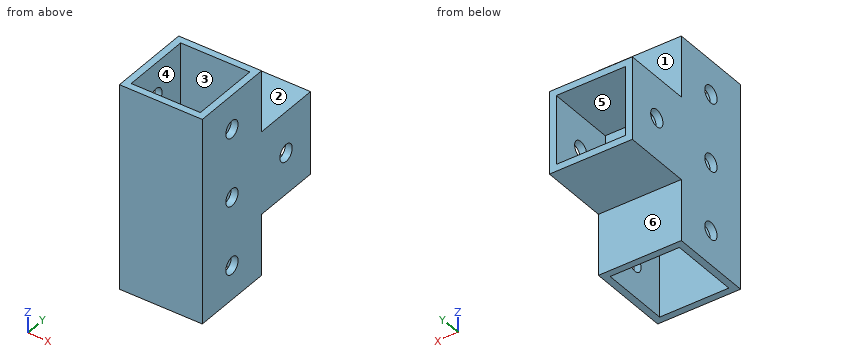
from build123d import *

# Parameters (mm, degrees)
SKETCH_2_W          = 24.2
SKETCH_2_H          = 24.2
SKETCH_2_W_2        = 20.2
SKETCH_2_H_2        = 20.2
EXTRUDE_4_DEPTH     = 100
SKETCH_6_W          = 24.2
SKETCH_6_H          = 24.2
SKETCH_6_W_2        = 20.2
SKETCH_6_H_2        = 20.2
EXTRUDE_5_DEPTH     = 40
SKETCH_7_R          = 2.5
CUT_EXTRUDE_1_DEPTH = 40
SKETCH_8_R          = 2.5
CUT_EXTRUDE_2_DEPTH = 40
CUT_EXTRUDE_START   = -40
SKETCH_9_W          = 20
SKETCH_9_H          = 24.2
SKETCH_9_R          = 2.5
CUT_EXTRUDE_3_DEPTH = 40
SKETCH_10_W         = 24.2
SKETCH_10_H         = 20
SKETCH_10_R         = 2.5
CUT_EXTRUDE_4_DEPTH = 40


with BuildPart() as part:
    # 草图2 → 凸台-拉伸4 (new body)
    with BuildSketch(Plane.XY):
        Rectangle(SKETCH_2_W, SKETCH_2_H)
        Rectangle(SKETCH_2_W_2, SKETCH_2_H_2, mode=Mode.SUBTRACT)
    extrude(amount=EXTRUDE_4_DEPTH)

    # 草图6 → 凸台-拉伸5 (add)
    with BuildSketch(Plane(origin=(0, 12.1, 0), x_dir=(1, 0, 0), z_dir=(0, 1, 0))):
        with Locations((0, -50)):
            Rectangle(SKETCH_6_W, SKETCH_6_H)
        with Locations((0, -50)):
            Rectangle(SKETCH_6_W_2, SKETCH_6_H_2, mode=Mode.SUBTRACT)
    extrude(amount=EXTRUDE_5_DEPTH)

    # 草图7 → 切除-拉伸1 (cut)
    with BuildSketch(Plane.ZY.offset(12.1)):
        with Locations((10, 0)):
            Circle(SKETCH_7_R)
        with Locations((30, 0)):
            Circle(SKETCH_7_R)
        with Locations(Location((90, 0, 0), (0, 0, 180))):
            Circle(SKETCH_7_R)
        with Locations(Location((70, 0, 0), (0, 0, 180))):
            Circle(SKETCH_7_R)
        with Locations((50, 42.1)):
            Circle(SKETCH_7_R)
        with Locations((50, 22.1)):
            Circle(SKETCH_7_R)
    extrude(amount=-CUT_EXTRUDE_1_DEPTH, mode=Mode.SUBTRACT)

    # 草图8 → 切除-拉伸2 (cut)
    with BuildSketch(Plane(origin=(12.1, 0, 0), x_dir=(0, 0, -1), z_dir=(1, 0, 0))):
        with Locations((-50, 0)):
            Circle(SKETCH_8_R)
    extrude(amount=-CUT_EXTRUDE_2_DEPTH, mode=Mode.SUBTRACT)

    # 草图9 → 切除-拉伸3 (cut)
    # profile 1 of 2: a face of its own
    with BuildSketch(Plane(origin=(12.1, 0, 0), x_dir=(0, 0, -1), z_dir=(1, 0, 0)).offset(CUT_EXTRUDE_START)):
        with Locations((-10, 0)):
            Rectangle(SKETCH_9_W, SKETCH_9_H)
        with Locations((-10, 0)):
            Circle(SKETCH_9_R, mode=Mode.SUBTRACT)
    # profile 2 of 2: a face of its own
    with BuildSketch(Plane(origin=(12.1, 0, 0), x_dir=(0, 0, -1), z_dir=(1, 0, 0)).offset(CUT_EXTRUDE_START)):
        with Locations((-90, 0)):
            Rectangle(SKETCH_9_W, SKETCH_9_H)
        with Locations((-90, 0)):
            Circle(SKETCH_9_R, mode=Mode.SUBTRACT)
    extrude(amount=CUT_EXTRUDE_3_DEPTH, mode=Mode.SUBTRACT)

    # 草图10 → 切除-拉伸4 (cut)
    with BuildSketch(Plane(origin=(12.1, 0, 0), x_dir=(0, 0, -1), z_dir=(1, 0, 0)).offset(CUT_EXTRUDE_START)):
        with Locations((-50, 42.1)):
            Rectangle(SKETCH_10_W, SKETCH_10_H)
        with Locations((-50, 42.1)):
            Circle(SKETCH_10_R, mode=Mode.SUBTRACT)
    extrude(amount=CUT_EXTRUDE_4_DEPTH, mode=Mode.SUBTRACT)


solid = part.part
Source: CAD feature listing. Evaluate the final solid. Frame: model axes, mm. Face numbers are marked on the shaded views. A direction names the side the tool comes from. Round coordinates to 2 decimals unless told otherwise and drop trailing zeros. Write each loop counter-clockwise with the first axis right and the second up, starting at its lowest first coordinate (ties: lowest second). Pieces come first, ordered by that corner, then holes. Notation, with made-up numbers: M -20.5,-15 L 8.5,-15 A18 ccw 8.5,-1 Z; hole C 42,83.25 d6. An arc over 180 degrees is marked long. One line per item, written item: value. Start each with the question number.
Item 1: Section query A-A (y = 0). State how many separate pieces and enclosed holes the cut face has, plus the area to 3 significant figures.
Item 2: Ray query, L1, parallel to Y at x = -1.75, z = 65.5; L2, parallel to Y at x = 10.95, z = 70; L3, parallel to Y at x = -10.6, z = 50. Return the intervals inside material, ascending. Write a range as from..to.
Item 3: Section query B-B (z = 50). Return the cut outline in (x, y).
Item 4: Mould query, pull axis Y, two halves, no side actions, for the marked faces 1, 2 and 3. Classes: pulls with the +Y half, pulls with the -Y half, needs draft (parallel to the pull), parting line crosses it, or undercut.
Item 5: Pin query (flat end, axial travel): pin 1 (6 mm diameter, centred on x = -5.5, y = 6, fed in from -Z); pin 2 (14.5 mm diameter, centred on x = 4.5, z = 30.5, fed in from +Y); pin 3 (6 mm diameter, centred on x = 0.5, y = 24, fed in from +Z); pin 4 (10 mm diameter, centred on x = 0.5, y = 25.5, fed in from -Z). Return the tip coordinate at first contact, or that it passes through.
Item 6: Section query D-D (y = 22.1). Return the cut outline in (x, z).
Item 7: Section query C-C (x = -6). Return the cut outline in (y, z), plus the area to 3 significant figures.
Item 8: Set-up query: the marked faces 4, 5 and 6. Return all of +Z, -Z, +X, -X, +Y, -Y with unobstructed straight access to the full face (end or side cutting, diameter ignored); none if empty.
Result set:
1. separate pieces: 8
1. enclosed holes: 0
1. area: 180 mm²
2. L1: y = -12.1..-10.1, 10.1..12.1
2. L2: y = -12.1..-2.5, 2.5..12.1
2. L3: y = -12.1..-2.5, 2.5..19.6, 24.6..32.1
3. outline: M -12.1,-12.1 L 12.1,-12.1 L 12.1,-2.5 L 10.1,-2.5 L 10.1,-10.1 L -10.1,-10.1 L -10.1,-2.5 L -12.1,-2.5 Z; M -12.1,2.5 L -10.1,2.5 L -10.1,10.1 L 10.1,10.1 L 10.1,2.5 L 12.1,2.5 L 12.1,19.6 L 10.1,19.6 L 10.1,12.1 L -10.1,12.1 L -10.1,19.6 L -12.1,19.6 Z; M -12.1,24.6 L -10.1,24.6 L -10.1,32.1 L -12.1,32.1 Z; M 10.1,24.6 L 12.1,24.6 L 12.1,32.1 L 10.1,32.1 Z
4. face 1: pulls with the +Y half
4. face 2: needs draft
4. face 3: undercut
5. pin 1: passes through
5. pin 2: stops at y = 12.1
5. pin 3: stops at z = 62.1
5. pin 4: stops at z = 37.9
6. outline: M -12.1,37.9 L 12.1,37.9 L 12.1,47.5 L 10.1,47.5 L 10.1,39.9 L -10.1,39.9 L -10.1,47.5 L -12.1,47.5 Z; M -12.1,52.5 L -10.1,52.5 L -10.1,60.1 L 10.1,60.1 L 10.1,52.5 L 12.1,52.5 L 12.1,62.1 L -12.1,62.1 Z
7. outline: M -12.1,20 L -10.1,20 L -10.1,80 L -12.1,80 Z; M 10.1,20 L 12.1,20 L 12.1,37.9 L 32.1,37.9 L 32.1,39.9 L 12.1,39.9 L 12.1,60.1 L 32.1,60.1 L 32.1,62.1 L 12.1,62.1 L 12.1,80 L 10.1,80 Z
7. area: 320 mm²
8. face 4: +Z, -Z
8. face 5: +Y
8. face 6: -Z, +X, -X, +Y
